Part model, mm, in its own coordinate system. A direction names the side the tool comes from. Give positions to 0.01 mm unless a question says otherwise; leave off trailing zeros. Order: outer loops, then holes, each group sorted by start corner. A loop starts at its lowest first (then second) coordinate and runs counter-clockwise, first axis right, second up. Notation, with made-up numbers: (-36, 7) - (20, 7) arc R21 ccw to (20, 29) - close; hole circle Ø9 at (-12, 22.5). An arc over 180 degrees is marked (long way). One line per item, written item: value.
```python
from build123d import *

# Parameters (mm, degrees)
SKETCH1_W           = 80
SKETCH1_H           = 80
SKETCH1_R           = 5
BOSS_EXTRUDE1_DEPTH = 5
SKETCH2_R           = 7.5
SKETCH2_R_2         = 5
EXTRUDE_THIN1_DEPTH = 5
SKETCH3_R           = 2
CUT_EXTRUDE1_DEPTH  = 11
FILLET1_R           = 5


with BuildPart() as part:
    # Sketch1 → Boss-Extrude1 (new body)
    with BuildSketch(Plane(origin=(0, 0, 0), x_dir=(1, 0, 0), z_dir=(0, 1, 0))):
        Rectangle(SKETCH1_W, SKETCH1_H)
        with Locations((-30, 30)):
            Circle(SKETCH1_R, mode=Mode.SUBTRACT)
        with Locations((30, 30)):
            Circle(SKETCH1_R, mode=Mode.SUBTRACT)
        with Locations((30, -30)):
            Circle(SKETCH1_R, mode=Mode.SUBTRACT)
        with Locations((-30, -30)):
            Circle(SKETCH1_R, mode=Mode.SUBTRACT)
    extrude(amount=BOSS_EXTRUDE1_DEPTH)

    # Sketch2 → Extrude-Thin1 (add)
    with BuildSketch(Plane.XZ):
        with Locations((-30, -30)):
            Circle(SKETCH2_R)
        with Locations((-30, -30)):
            Circle(SKETCH2_R_2, mode=Mode.SUBTRACT)
        with Locations((30, -30)):
            Circle(SKETCH2_R)
        with Locations((30, -30)):
            Circle(SKETCH2_R_2, mode=Mode.SUBTRACT)
        with Locations((30, 30)):
            Circle(SKETCH2_R)
        with Locations((30, 30)):
            Circle(SKETCH2_R_2, mode=Mode.SUBTRACT)
        with Locations((-30, 30)):
            Circle(SKETCH2_R)
        with Locations((-30, 30)):
            Circle(SKETCH2_R_2, mode=Mode.SUBTRACT)
    extrude(amount=EXTRUDE_THIN1_DEPTH)

    # Sketch3 → Cut-Extrude1 (cut, through all)
    with BuildSketch(Plane(origin=(0, 5, 0), x_dir=(1, 0, 0), z_dir=(0, 1, 0))):
        Circle(SKETCH3_R)
    extrude(amount=-CUT_EXTRUDE1_DEPTH, mode=Mode.SUBTRACT)

    # Fillet1
    fillet1_edges = [part.edges().sort_by_distance(p)[0] for p in [
        (40, 2.5, 40),
        (-40, 2.5, 40),
        (-40, 2.5, -40),
        (40, 2.5, -40),
    ]]
    fillet(fillet1_edges, radius=FILLET1_R)


solid = part.part
```
1) Slice it at A-A on y = -1.5. Write the cut outline in (x, z).
Answer:
outline: circle Ø15 at (-30, -30); circle Ø15 at (-30, 30); circle Ø15 at (30, -30); circle Ø15 at (30, 30); hole circle Ø10 at (-30, -30); hole circle Ø10 at (-30, 30); hole circle Ø10 at (30, -30); hole circle Ø10 at (30, 30)
2) Drop flat-ended pins along their axis: P1, Ø9, axis at x = 30, z = -30, coming from the -Y side; P2, Ø5, axis at x = 15, y = -0.5, coming from the +Z side; P3, Ø10, axis at x = 12, z = -10.5, coming from the -Y side. Give the stop position or say it passes through.
Answer:
P1: passes through
P2: stops at z = 40
P3: stops at y = 0
3) Wall check: line 1 along Z through (x, y) = (30, -1); line 2 along Z through (x, y) = (-30, 2.75); line 3 along X through (y, z) = (-4, -31.5). Give the ranges that are in metal, low to high. Write a range as [from, to].
Answer:
line 1: z = [-37.5, -35], [-25, -22.5], [22.5, 25], [35, 37.5]
line 2: z = [-40, -35], [-25, 25], [35, 40]
line 3: x = [-37.35, -34.77], [-25.23, -22.65], [22.65, 25.23], [34.77, 37.35]
4) Slice it at D-D on y = 3. Write the cut outline in (x, z).
Answer:
outline: (-40, -35) arc R5 ccw to (-35, -40) - (35, -40) arc R5 ccw to (40, -35) - (40, 35) arc R5 ccw to (35, 40) - (-35, 40) arc R5 ccw to (-40, 35) - close; hole circle Ø10 at (-30, -30); hole circle Ø10 at (-30, 30); hole circle Ø4 at (0, 0); hole circle Ø10 at (30, -30); hole circle Ø10 at (30, 30)
5) Which spindle directions (+Z, -Z, +X, -X, +Y, -Y) get a long thin tool onto all of the face, cutting with end or side? Do faces 1 (the face through (-31.63, -2.46, -37.32)), 2 (the face through (-34, 0, -33)). Say none if no direction does.
Answer:
face 1: -Y
face 2: +Y, -Y
6) Slice it at C-C on x = 0. Write the cut outline in (y, z), then the cut area to 3 significant figures.
Answer:
outline: (0, -40) - (5, -40) - (5, -2) - (0, -2) - close; (0, 2) - (5, 2) - (5, 40) - (0, 40) - close
area: 380 mm2
7) Two-plate mould, pull along X, no slides. Class faces 3 (the face through (0, 3, 2)), 4 (the face through (40, 2, 0)), 5 (the face through (-25, -5, 28)): pulls with the +X half, pulls with the -X half, needs draft (parallel to the pull), parting line crosses it, or undercut.
Answer:
face 3: undercut
face 4: pulls with the +X half
face 5: needs draft
8) Slice it at B-B on z = 30. Write the cut outline in (x, y).
Answer:
outline: (-40, 0) - (-37.5, 0) - (-37.5, -5) - (-35, -5) - (-35, 5) - (-40, 5) - close; (-25, -5) - (-22.5, -5) - (-22.5, 0) - (22.5, 0) - (22.5, -5) - (25, -5) - (25, 5) - (-25, 5) - close; (35, -5) - (37.5, -5) - (37.5, 0) - (40, 0) - (40, 5) - (35, 5) - close
